from build123d import *

# Parameters (mm, degrees)
SKETCH1_R           = 14
BOSS_EXTRUDE1_DEPTH = 1
SKETCH2_R           = 11.875
BOSS_EXTRUDE2_DEPTH = 11
SKETCH3_R           = 14
BOSS_EXTRUDE3_DEPTH = 1
SKETCH4_R           = 9
BOSS_EXTRUDE4_DEPTH = 10
SKETCH5_R           = 2.5
CUT_EXTRUDE1_DEPTH  = 31.347981811


with BuildPart() as part:
    # Sketch1 → Boss-Extrude1 (new body)
    with BuildSketch(Plane(origin=(0, 0, 0), x_dir=(0, 0, -1), z_dir=(1, 0, 0))):
        Circle(SKETCH1_R)
    extrude(amount=BOSS_EXTRUDE1_DEPTH)

    # Sketch2 → Boss-Extrude2 (add)
    with BuildSketch(Plane(origin=(1, 0, 0), x_dir=(0, 0, -1), z_dir=(1, 0, 0))):
        Circle(SKETCH2_R)
    extrude(amount=BOSS_EXTRUDE2_DEPTH)

    # Sketch3 → Boss-Extrude3 (add)
    with BuildSketch(Plane(origin=(12, 0, 0), x_dir=(0, 0, -1), z_dir=(1, 0, 0))):
        Circle(SKETCH3_R)
    extrude(amount=BOSS_EXTRUDE3_DEPTH)

    # Sketch4 → Boss-Extrude4 (add)
    with BuildSketch(Plane(origin=(13, 0, 0), x_dir=(0, 0, -1), z_dir=(1, 0, 0))):
        Circle(SKETCH4_R)
    extrude(amount=BOSS_EXTRUDE4_DEPTH)

    # Sketch5 → Cut-Extrude1 (cut, through all)
    with BuildSketch(Plane(origin=(23, 0, 0), x_dir=(0, 0, -1), z_dir=(1, 0, 0))):
        Circle(SKETCH5_R)
    extrude(amount=-CUT_EXTRUDE1_DEPTH, mode=Mode.SUBTRACT)


solid = part.part
Geometry check sheet. Reference: the model listing, model coordinates, mm. A direction names the side the tool comes from. Coordinates: 2 decimals unless noted, no trailing zeros. Order: outer loops, then holes, each group sorted by start corner. A loop starts at its lowest first (then second) coordinate and runs counter-clockwise, first axis right, second up. Notation, with made-up numbers: (31, -3.75) - (51, -3.75) arc R9 cw to (51, 10.25) - close; hole circle Ø6 at (-40, 9.5). An arc over 180 degrees is marked (long way). Answer in a Markdown table with one row per item. Add a question column.
1) Material ranges on line 1 along Y through (x, z) = (9.25, 0) (3 decimals); line 2 along Y through (x, z) = (15, 0); line 3 along X through (y, z) = (-8.75, -5.5), recorded low to high. Write a range as [from, to].
2) Release check for a two-part mould opening along X. For faces 1 (the flat face through (1, -10.3, 6.3)), 2 (the cylindrical face through (17.93, 8.923, 1.172)), 3 (the flat face through (13, -9, -3)) record: +X half, -X half, draft (parallel to the pull), parting line (faces both ways), or undercut.
3) Cross-section at C-C, the plane x = 19. Record the cut outline in (y, z).
4) Gauge pin test, flat ends, axial feed: P1, Ø4, axis at y = -4, z = 10.5, coming from the +X side; P2, Ø2, axis at x = 8.5, z = -3, coming from the +Y side; P3, Ø8, axis at x = 8.5, z = -4.5, coming from the +Y side. Record the tip position at first contact, or that the pin passes through.
5) Cross-section at D-D, the plane z = -8. Record the cut outline in (x, y).
6) Set-up check for faces 4 (the flat face through (12, -10.3, 6.3)), 5 (the cylindrical face through (11.66, -2.44, 0.54)): record each of +Z, -Z, +X, -X, +Y, -Y from which the full face is reachable in a straight line by a thin tool's end or side.
7) Cross-section at A-A, the plane y = 0. Record the cut outline in (x, z) (3 decimals).
Check result:
| question | item | result |
|---|---|---|
| 1 | line 1 | y = [-11.875, -2.5], [2.5, 11.875] |
| 1 | line 2 | y = [-9, -2.5], [2.5, 9] |
| 1 | line 3 | x = [0, 13] |
| 2 | face 1 | undercut |
| 2 | face 2 | draft |
| 2 | face 3 | +X half |
| 3 | outline | circle Ø18 at (0, 0); hole circle Ø5 at (0, 0) |
| 4 | P1 | stops at x = 13 |
| 4 | P2 | stops at y = 11.71 |
| 4 | P3 | stops at y = 13.76 |
| 5 | outline | (0, -11.49) - (1, -11.49) - (1, -8.78) - (12, -8.78) - (12, -11.49) - (13, -11.49) - (13, -4.12) - (23, -4.12) - (23, 4.12) - (13, 4.12) - (13, 11.49) - (12, 11.49) - (12, 8.78) - (1, 8.78) - (1, 11.49) - (0, 11.49) - close |
| 6 | face 4 | none |
| 6 | face 5 | +X, -X |
| 7 | outline | (0, -14) - (1, -14) - (1, -11.875) - (12, -11.875) - (12, -14) - (13, -14) - (13, -9) - (23, -9) - (23, -2.5) - (0, -2.5) - close; (0, 2.5) - (23, 2.5) - (23, 9) - (13, 9) - (13, 14) - (12, 14) - (12, 11.875) - (1, 11.875) - (1, 14) - (0, 14) - close |
